```python
from build123d import *


with BuildPart() as part:
    # Sketch1 → Revolve1 (revolve)
    with BuildSketch(Plane.XY, mode=Mode.PRIVATE) as revolve1_sk:
        Polygon((-1.9, 4), (-1.9, 0), (0, 0), (62.4, 0), (64.3, 0), (64.3, 4), (63.3, 4), (63.3, 3.8), (62.4, 3.8), (62.4, 4), (0, 4), (0, 3.8), (-0.9, 3.8), (-0.9, 4), align=None)
        Polygon((62.4, 1.680571503), (62.4, 1.781506728), (62.123398622, 1.781506728), align=None, mode=Mode.SUBTRACT)
    revolve(revolve1_sk.sketch.rotate(Axis((0, 0, 0), (1, 0, 0)), 90), axis=Axis((0, 0, 0), (1, 0, 0)))


solid = part.part
```
Part model, mm, in its own coordinate system. A direction names the side the tool comes from. Coordinates: 2 decimals unless noted, no trailing zeros. Loops run counter-clockwise (first coordinate to the right, second up) from the corner with the lowest first, then second, coordinate; pieces in that order, holes last. Notation, with made-up numbers: (17.25, 27) - (61.25, 27) arc R19 cw to (61.25, 46) - close; hole circle Ø11 at (77.25, 64). An arc over 180 degrees is marked (long way). Write item = value, one per line. Start each with the question number.
Item 1: Cut at B-B, the plane y = 3.25. Give the cut face in (x, z).
Item 2: Cut at A-A, the plane x = 50. Give the cut face in (y, z).
Item 3: Wall check: L1, parallel to X at y = 1, z = 3.75; L2, parallel to Y at x = 34, z = 3.25; L3, parallel to Z at x = 55, y = 0.5. Give the ranges that are in metal, low to high. Write a range as from..to.
Item 4: Flat gauge pin, fed straight in: pin 1 Ø2 at (x, z) = (30.5, 2) entering from +Y. Where does the tip first touch, or does it go through?
Item 5: Cut at D-D, the plane y = -3. Give the cut face in (x, z).
Item 6: 3-axis set-ups, long thin cutter, end or side, ignore diameter. For faces 1 (the cylindrical face through (62.844, -1.141, 3.625)), 2 (the flat face through (-1.9, 0, 0)): which of +Z, -Z, +X, -X, +Y, -Y reach the whole face in a straight line?
Item 7: Cut at C-C, the plane z = 1. State how many separate pieces and enclosed holes the cut face has, and give its area (3 significant figures).
The answers:
q1.outline = (-1.9, -2.33) - (-0.9, -2.33) - (-0.9, -1.97) - (0, -1.97) - (0, -2.33) - (62.4, -2.33) - (62.4, -1.97) - (63.3, -1.97) - (63.3, -2.33) - (64.3, -2.33) - (64.3, 2.33) - (63.3, 2.33) - (63.3, 1.97) - (62.4, 1.97) - (62.4, 2.33) - (0, 2.33) - (0, 1.97) - (-0.9, 1.97) - (-0.9, 2.33) - (-1.9, 2.33) - close
q2.outline = circle Ø8 at (0, 0)
q3.L1 = -1.9..-0.9, 0..62.4, 63.3..64.3
q3.L2 = -2.33..2.33
q3.L3 = -3.97..3.97
q4.pin_1 = 3.87
q5.outline = (-1.9, -2.65) - (-0.9, -2.65) - (-0.9, -2.33) - (0, -2.33) - (0, -2.65) - (62.4, -2.65) - (62.4, -2.33) - (63.3, -2.33) - (63.3, -2.65) - (64.3, -2.65) - (64.3, 2.65) - (63.3, 2.65) - (63.3, 2.33) - (62.4, 2.33) - (62.4, 2.65) - (0, 2.65) - (0, 2.33) - (-0.9, 2.33) - (-0.9, 2.65) - (-1.9, 2.65) - close
q6.face_1 = none
q6.face_2 = +Z, -Z, -X, +Y, -Y
q7.separate_pieces = 1
q7.enclosed_holes = 2
q7.area = 512 mm2
